from build123d import *

# Parameters (mm, degrees)
SKETCH1_R           = 6.25
BOSS_EXTRUDE1_DEPTH = 16.5
CUT_EXTRUDE1_REACH  = 20.718
SKETCH2_W           = 5.5
SKETCH2_H           = 5.5
SKETCH3_R           = 12.5
BOSS_EXTRUDE2_DEPTH = 4
FILLET1_R           = 1
SKETCH4_W           = 0.5
SKETCH4_H           = 30
CUT_EXTRUDE2_DEPTH  = 0.5


with BuildPart() as part:
    # Sketch1 → Boss-Extrude1 (new body)
    with BuildSketch(Plane(origin=(0, 0, 0), x_dir=(1, 0, 0), z_dir=(0, 1, 0))):
        with Locations(Location((0, 0, 0), (0, 0, 270))):
            Circle(SKETCH1_R)
    extrude(amount=BOSS_EXTRUDE1_DEPTH)

    # Sketch2 → Cut-Extrude1 (cut, up to next)
    with BuildSketch(Plane(origin=(0, 16.5, 0), x_dir=(1, 0, 0), z_dir=(0, 1, 0)), mode=Mode.PRIVATE) as cut_extrude1_sk1:
        with Locations((0, -6.5)):
            Rectangle(SKETCH2_W, SKETCH2_H)
    cut_extrude1_tool1 = extrude(cut_extrude1_sk1.sketch, amount=-CUT_EXTRUDE1_REACH, mode=Mode.PRIVATE) & part.part
    add(cut_extrude1_tool1.solids().sort_by_distance((0, 16.5, 6.5))[0], mode=Mode.SUBTRACT)

    # Sketch3 → Boss-Extrude2 (add)
    with BuildSketch(Plane(origin=(0, 16.5, 0), x_dir=(1, 0, 0), z_dir=(0, 1, 0))):
        with Locations(Location((0, 0, 0), (0, 0, 270))):
            Circle(SKETCH3_R)
    extrude(amount=BOSS_EXTRUDE2_DEPTH)

    # Fillet1
    fillet1_edges = [part.edges().sort_by_distance(p)[0] for p in [
        (0, 20.5, -12.5),
    ]]
    fillet(fillet1_edges, radius=FILLET1_R)

    # Sketch4 → Cut-Extrude2 (cut)
    with BuildSketch(Plane(origin=(0, 20.5, 0), x_dir=(1, 0, 0), z_dir=(0, 1, 0))):
        Rectangle(SKETCH4_W, SKETCH4_H)
        with Locations((2, 0)):
            Rectangle(SKETCH4_W, SKETCH4_H)
        with Locations((-2, 0)):
            Rectangle(SKETCH4_W, SKETCH4_H)
    extrude(amount=-CUT_EXTRUDE2_DEPTH, mode=Mode.SUBTRACT)


solid = part.part
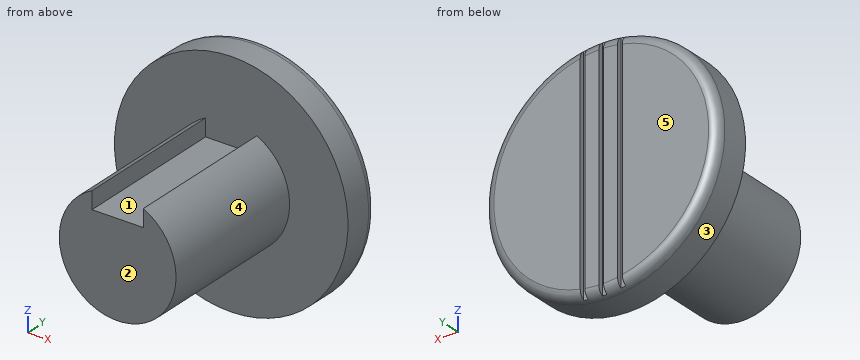
Design review of the part built by this model. Coordinates are the model's own, in mm. Face numbers are marked on the shaded views. A direction names the side the tool comes from. Coordinates: 2 decimals unless noted, no trailing zeros. Loops run counter-clockwise (first coordinate to the right, second up) from the corner with the lowest first, then second, coordinate; pieces in that order, holes last. Notation, with made-up numbers: (31, 10.25) - (71, 10.25) arc R26 ccw to (71, 48.25) - close; hole circle Ø9 at (27.5, 44.5). An arc over 180 degrees is marked (long way). Use CSV: the item, a comma, the result in double quotes. Start each with the question number.
1. To check wall thickness, follow probe 1 along Y at (x, z) = (-5, -8.25); probe 2 along Z at (x, y) = (3.75, 11); probe 3 along X at (y, z) = (1.5, -5.25). State the ranges of each line that lie inside material, in increasing order.
2. Mouldability with a two-part tool opening along X and no side actions: class the marked faces 1, 2 and 3 as released by +X, released by -X, zero draft, split by the parting line, or undercut.
3. Add section B-B on y = 15.5. Give the boundary of the cut face in (x, z).
4. Add section A-A on z = 0. Give the boundary of the cut face in (x, y).
5. For the marked faces 4 and 5, list the 3-axis set-ups (+Z, -Z, +X, -X, +Y, -Y) from which the entire face can be reached by the end or side of a thin tool; tool diameter is ignored.
6. Clearance check with flat-ended pins moving along their axes: pin 1 (4 mm diameter, centred on y = 11, z = 6, fed in from +X); pin 2 (0.9 mm diameter, centred on y = 7, z = 4, fed in from +X); pin 3 (3 mm diameter, centred on x = -6.5, y = 16, fed in from -Z). State where each tip first meets the part, or that it passes through.
Resolved:
1,probe 1,"16.5 to 20.5"
1,probe 2,"-5 to 5"
1,probe 3,"-3.39 to 3.39"
2,face 1,"undercut"
2,face 2,"zero draft"
2,face 3,"split by the parting line"
3,outline,"(-2.75, 3.75) - (-2.75, 5.61) arc R6.25 ccw (long way) to (2.75, 5.61) - (2.75, 3.75) - close"
4,outline,"(-12.5, 16.5) - (-6.25, 16.5) - (-6.25, 0) - (6.25, 0) - (6.25, 16.5) - (12.5, 16.5) - (12.5, 19.5) arc R1 ccw to (11.5, 20.5) - (2.25, 20.5) - (2.25, 20) - (1.75, 20) - (1.75, 20.5) - (0.25, 20.5) - (0.25, 20) - (-0.25, 20) - (-0.25, 20.5) - (-1.75, 20.5) - (-1.75, 20) - (-2.25, 20) - (-2.25, 20.5) - (-11.5, 20.5) arc R1 ccw to (-12.5, 19.5) - close"
5,face 4,"-Y"
5,face 5,"+Z, -Z, +X, -X, +Y"
6,pin 1,"x = 4.8"
6,pin 2,"x = 5.14"
6,pin 3,"z = -11.42"
